Can you work these out from the model? Positions are in its coordinate system, mm. A direction names the side the tool comes from. Give positions to 0.01 mm unless a question says otherwise; leave off trailing zeros. Write each loop counter-clockwise with the first axis right and the second up, starting at its lowest first coordinate (ties: lowest second). Pieces come first, ordered by that corner, then holes. Notation, with made-up numbers: M 59.25,56 L 74.25,56 A35 ccw 74.25,94 Z; hole C -14.5,64.25 d9. An arc over 180 degrees is marked long. Answer as CSV lines item,"result". Start each with the question number.
Solid Edge part; units mm, degrees
sketch "Sketch1" plane through (-41.275, 0, 0) normal (1, 0, 0) x (0, 1, 0)
  circle A0 centre (-29.2392, 18.9195) radius 15
extrude "ExtrudedProtrusion_1" add sketch "Sketch1" along normal blind 80
fillet "Round_1" radius 1 1 edges at (38.725, -44.2392, 18.9195)
fillet "Round_2" radius 5 1 edges at (-41.275, -44.2392, 18.9195)
sketch "Sketch2" plane through (-41.275, -29.2392, 18.9195) normal (-1, 0, 0) x (0, 0, -1)
  circle A0 centre (0, 0) radius 8
extrude "ExtrudedProtrusion_2" add sketch "Sketch2" along normal blind 40
sketch "Sketch3" plane through (0, 0, 32) normal (0, 0, 1) x (1, 0, 0)
  circle A0 centre (-31.0799, -29.2392) radius 1.75
extrude "ExtrudedProtrusion_3" add sketch "Sketch3" along normal blind 5
sketch "Sketch4" plane through (38.725, -29.2392, 18.9195) normal (1, 0, 0) x (0, 1, 0)
  circle A0 centre (0, 11.3356) radius 1.75
extrude "ExtrudedProtrusion_4" add sketch "Sketch4" along normal blind 3.5
sketch "Sketch5" plane through (0, 0, 0) normal (0, 0, 1) x (1, 0, 0)
  circle A0 centre (32.725, -10.2392) radius 2
  circle A1 centre (32.725, -48.2392) radius 2
  line L0 (-20.775, -5.2392) -> (-13.775, -5.2392)
  arc A2 (-13.775, -5.2392) -> (-12.275, -6.7392) centre (-13.775, -6.7392) cw
  line L1 (-12.275, -6.7392) -> (-12.275, -51.7392)
  arc A3 (-12.275, -51.7392) -> (-13.775, -53.2392) centre (-13.775, -51.7392) cw
  line L2 (-13.775, -53.2392) -> (-20.775, -53.2392)
  arc A4 (-20.775, -53.2392) -> (-22.275, -51.7392) centre (-20.775, -51.7392) cw
  line L3 (-22.275, -51.7392) -> (-22.275, -6.7392)
  arc A5 (-22.275, -6.7392) -> (-20.775, -5.2392) centre (-20.775, -6.7392) cw
  circle A6 centre (-17.275, -10.2392) radius 2
  circle A7 centre (-17.275, -48.2392) radius 2
  line L4 (29.225, -5.2392) -> (36.225, -5.2392)
  arc A8 (36.225, -5.2392) -> (37.725, -6.7392) centre (36.225, -6.7392) cw
  line L5 (37.725, -6.7392) -> (37.725, -51.7392)
  arc A9 (37.725, -51.7392) -> (36.225, -53.2392) centre (36.225, -51.7392) cw
  line L6 (36.225, -53.2392) -> (29.225, -53.2392)
  arc A10 (29.225, -53.2392) -> (27.725, -51.7392) centre (29.225, -51.7392) cw
  line L7 (27.725, -51.7392) -> (27.725, -6.7392)
  arc A11 (27.725, -6.7392) -> (29.225, -5.2392) centre (29.225, -6.7392) cw
  dimension "D1" = 37.725
  dimension "D2" = 29.225
  dimension "D3" = 17.275
  dimension "D4" = 17.275
extrude "ExtrudedProtrusion_5" add sketch "Sketch5" along normal blind 2.5
sketch "Sketch6" plane through (43.6955, -29.1968, 2.5) normal (0, 0, 1) x (0, 1, 0)
  line L0 (-14, 13.5) -> (14, 13.5)
  line L1 (14, 13.5) -> (14, 15)
  line L2 (14, 15) -> (-14, 15)
  line L3 (-14, 15) -> (-14, 13.5)
  line L4 (-14.0424, 61.11) -> (13.9576, 61.11)
  line L5 (13.9576, 61.11) -> (13.9576, 62.61)
  line L6 (13.9576, 62.61) -> (-14.0424, 62.61)
  line L7 (-14.0424, 62.61) -> (-14.0424, 61.11)
extrude "Protrusion1" add sketch "Sketch6" along normal up to vertex (16.4195 mm away)
sketch "Sketch7" plane through (-81.275, -29.2392, 18.9195) normal (-1, 0, 0) x (0, 0, 1)
  circle A0 centre (0, 0) radius 8.835
extrude "ExtrudedProtrusion_7" add sketch "Sketch7" along normal blind 2
sketch "Sketch8" plane through (0, 0, 18.9195) normal (0, 0, 1) x (1, 0, 0)
  circle A0 centre (-92.6361, -29.2392) radius 2.5
  line L0 (-92.6361, -24.2392) -> (-83.275, -24.2392)
  line L1 (-83.275, -24.2392) -> (-83.275, -34.2392)
  line L2 (-92.6361, -34.2392) -> (-83.275, -34.2392)
  arc A1 (-92.6361, -34.2392) -> (-92.6361, -24.2392) centre (-92.6361, -29.2392) cw
extrude "ExtrudedProtrusion_8" add sketch "Sketch8" along normal mid plane 5
1) I want a section at B-B, the plane x = -27.5. Please give me the cut outline in (y, z).
2) I'm going to push flat-ended pins straight in: P1, Ø2.5, axis at x = -89, z = 19, coming from the +Y side; P2, Ø4, axis at y = -41, z = 20, coming from the +X side (3 decimals); P3, Ø1.2, axis at y = -32, z = 1, coming from the +X side (3 decimals); P4, Ø3, axis at x = 32.72, y = -48.24, coming from the +Z side. Where does each tip first touch, or does it pass through?
3) On a 3-axis mill with a long thin cutter (end or side, diameter ignored), from which of +Z, -Z, +X, -X, +Y, -Y can I reach the whole of each face in a straight line? I mean faces 5 (the cylindrical face through (40.45, -30.988, 30.178)), 6 (the flat face through (-89, -29, 16.42)), 7 (the flat face through (-88, -34.239, 19)). Say none if no direction works.
4) I need wall thicknesses on L1, parallel to X at y = -43, z = 6.5; L2, parallel to Y at x = -83.5, z = 20.5; L3, parallel to X at y = -34, z = 23.5 (3 decimals). Which ranges of each line are inside material? Lowest first, please. Write a range as from..to.
5) I want a section at A-A, the plane x = -86.5. Please give me the cut outline in (y, z), then the cut area to 3 significant figures.
6) Thinking about a two-plate mould opening in X: for faces 1 (the flat face through (-12.275, -29, 1)), 2 (the flat face through (-41.275, -36, 14)), 3 (the flat face through (30.196, -28.2, 3.5)), 4 (the flat face through (-31, -29, 37)), which applies, released by +X, released by -X, zero draft, split by the parting line, or undercut?
Values found:
1,outline,"C -29.24,18.92 d30"
2,P1,"stops at y = -24.24"
2,P2,"stops at x = 38.725"
2,P3,"stops at x = 37.725"
2,P4,"passes through"
3,face 5,"+X"
3,face 6,"-Z, -X, +Y, -Y"
3,face 7,"+Z, -Z, -X, -Y"
4,L1,"x = -18.91..-17.41, 28.7..30.2"
4,L2,"y = -34.24..-24.24"
4,L3,"x = -83.275..38.725"
5,outline,"M -34.24,16.42 L -24.24,16.42 L -24.24,21.42 L -34.24,21.42 Z"
5,area,"50.0 mm²"
6,face 1,"undercut"
6,face 2,"undercut"
6,face 3,"released by +X"
6,face 4,"zero draft"
